The drawing under review shows one solid part. Ordinate dimensions are in mm from its lowest x, y, z. Coordinates: 2 decimals unless noted, no trailing zeros. Order: outer loops, then holes, each group sorted by start corner. A loop starts at its lowest first (then second) coordinate and runs counter-clockwise, first axis right, second up. Notation, with made-up numbers: (77, 87.25) - (129, 87.25) arc R21 ccw to (129, 98.25) - close; hole circle Ø9 at (28, 80.25). An arc over 180 degrees is marked (long way). Answer in a Markdown table with one row per item.
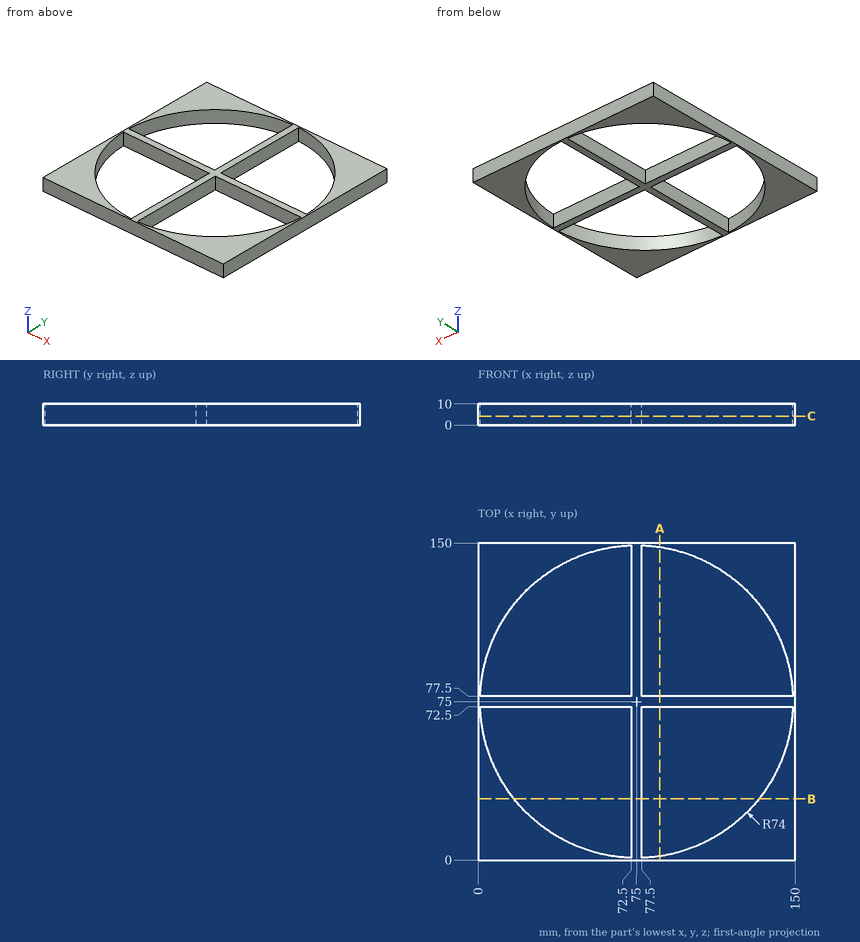
Item 1: To check wall thickness, follow line 1 (X direction, y = 62, z = 3); line 2 (Y direction, x = 112, z = 9); line 3 (X direction, y = 33, z = 8). State the ranges of each line that lie inside material, in increasing order. Write a range as from..to.
Check values:
| item | result |
|---|---|
| line 1 | 0..2.15, 72.5..77.5, 147.85..150 |
| line 2 | 0..10.91, 72.5..77.5, 139.09..150 |
| line 3 | 0..14.07, 72.5..77.5, 135.93..150 |
Item 2: We need section B-B, the plane y = 29. Write out the cut boundary in (x, z).
Check values:
| item | result |
|---|---|
| outline | (0, 0) - (17.03, 0) - (17.03, 10) - (0, 10) - close; (72.5, 0) - (77.5, 0) - (77.5, 10) - (72.5, 10) - close; (132.97, 0) - (150, 0) - (150, 10) - (132.97, 10) - close |
Item 3: We need section A-A, the plane x = 86. Write out the cut boundary in (y, z).
Check values:
| item | result |
|---|---|
| outline | (0, 0) - (1.82, 0) - (1.82, 10) - (0, 10) - close; (72.5, 0) - (77.5, 0) - (77.5, 10) - (72.5, 10) - close; (148.18, 0) - (150, 0) - (150, 10) - (148.18, 10) - close |
Item 4: We need section C-C, the plane z = 4.25. Write out the cut boundary in (x, y), then the cut area to 3 significant figures.
Check values:
| item | result |
|---|---|
| outline | (0, 0) - (150, 0) - (150, 150) - (0, 150) - close; hole (1.04, 72.5) arc R74 ccw to (72.5, 1.04) - (72.5, 72.5) - close; hole (1.04, 77.5) - (72.5, 77.5) - (72.5, 148.96) arc R74 ccw to start; hole (77.5, 1.04) arc R74 ccw to (148.96, 72.5) - (77.5, 72.5) - close; hole (77.5, 77.5) - (148.96, 77.5) arc R74 ccw to (77.5, 148.96) - close |
| area | 6,750 mm^2 |
